Can you work these out from the model? Positions are in its coordinate system, mm. Face numbers are marked on the shaded views. A direction names the side the tool comes from. Coordinates: 2 decimals unless noted, no trailing zeros. Write each loop counter-clockwise with the first axis right and the second up, starting at its lowest first coordinate (ties: lowest second). Pieces come first, ordered by that corner, then holes. Notation, with made-up numbers: (73, 13.5) - (82, 13.5) arc R32 ccw to (82, 51.5) - close; hole circle Ø9 at (-6.5, -11.75). An arc over 180 degrees is marked (long way). Use one line per item in the form item = value. Start each with the question number.
(1) On a 3-axis mill with a long thin cutter (end or side, diameter ignored), from which of +Z, -Z, +X, -X, +Y, -Y can I reach the whole of each face in a straight line? I mean the marked faces 1 and 2. Say none if no direction works.
(2) If I drill on probe 1 along X at (y, z) = (-45, -21); probe 2 along Y at (x, z) = (30.5, 37.5); probe 3 along Y at (x, z) = (116.5, -4), over which ranges is the centre line in solid material (lowest first)? Write a range as from..to.
(3) For pin 1 Ø12 at (y, z) = (-48.5, 40.5) entering from -X; pin 2 Ø10 at (x, z) = (-73.5, 34) entering from -Y; pin 3 Ø23 at (x, z) = (-11.28, 0) entering from -Y, each with a flat end and sliding along its axis, tell me the tip position at first contact or that it passes through.
(4) If we section it at C-C on x = -7: Please give me the cut outline in (y, z), then the cut area to 3 significant figures.
(5) If we section it at A-A on z = 0: Please give me the cut outline in (x, y).
(6) If we section it at D-D on z = 127: Please give me the cut outline in (x, y).
(7) If we section it at B-B on y = -76.5: Please give me the cut outline in (x, z).
```python
from build123d import *

# Parameters (mm, degrees)
F0_W     = 203.2
F0_H     = 304.8
F1_DEPTH = 25.4
F2_W     = 25.4
F2_H     = 304.8
F2_W_2   = 129.4638
F3_DEPTH = 25.4
F4_R     = 12.7
F5_DEPTH = 25.401
F6_R     = 11.1125
F7_DEPTH = 25.401


with BuildPart() as f1:
    # F0 (on Front) → F1 (new body)
    with BuildSketch(Plane.XZ):
        Rectangle(F0_W, F0_H)
    extrude(amount=-F1_DEPTH)

    # F2 (on face) → F3 (join)
    with BuildSketch(Plane.YZ.offset(101.6)):
        with Locations((12.7, 0)):
            Rectangle(F2_W, F2_H)
        with Locations((-64.7319, 0)):
            Rectangle(F2_W_2, F2_H)
    extrude(amount=F3_DEPTH)

    # F4 (on face) → F5 (cut, through all)
    with BuildSketch(Plane.XZ):
        with Locations((-11.2776, 0)):
            Circle(F4_R)
    extrude(amount=-F5_DEPTH, mode=Mode.SUBTRACT)

    # F6 (on face) → F7 (cut, through all)
    with BuildSketch(Plane(origin=(101.6, 0, 0), x_dir=(0, -1, 0), z_dir=(-1, 0, 0))):
        with Locations((69.3547, 0)):
            Circle(F6_R)
    extrude(amount=-F7_DEPTH, mode=Mode.SUBTRACT)


solid = f1.part
```
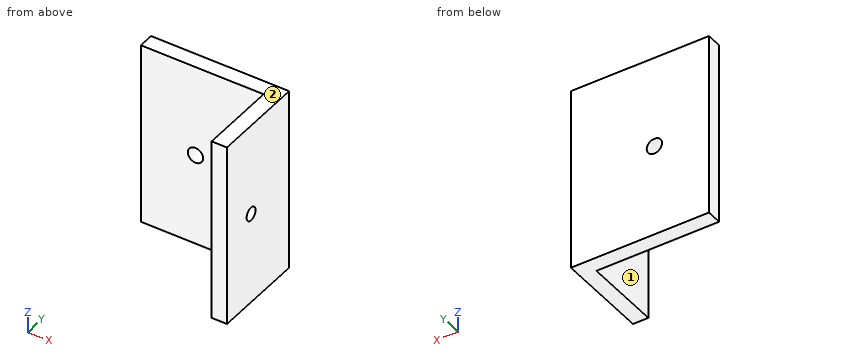
Reported:
q1.face_1 = +Z, -Z, -X, -Y
q1.face_2 = +Z, +X, -X, +Y, -Y
q2.probe_1 = 101.6..127
q2.probe_2 = 0..25.4
q2.probe_3 = -129.46..-79.72, -58.99..25.4
q3.pin_1 = 101.6
q3.pin_2 = 0
q3.pin_3 = through
q4.outline = (0, -152.4) - (25.4, -152.4) - (25.4, -11.96) - (0, -11.96) - close; (0, 11.96) - (25.4, 11.96) - (25.4, 152.4) - (0, 152.4) - close
q4.area = 7,130 mm2
q5.outline = (-101.6, 0) - (-23.98, 0) - (-23.98, 25.4) - (-101.6, 25.4) - close; (1.42, 0) - (101.6, 0) - (101.6, -58.24) - (127, -58.24) - (127, 25.4) - (1.42, 25.4) - close; (101.6, -129.46) - (127, -129.46) - (127, -80.47) - (101.6, -80.47) - close
q6.outline = (-101.6, 0) - (101.6, 0) - (101.6, -129.46) - (127, -129.46) - (127, 25.4) - (-101.6, 25.4) - close
q7.outline = (101.6, -152.4) - (127, -152.4) - (127, -8.51) - (101.6, -8.51) - close; (101.6, 8.51) - (127, 8.51) - (127, 152.4) - (101.6, 152.4) - close
